```python
from build123d import *

# Parameters (mm, degrees)
SKETCH_5_W               = 17.572810229
SKETCH_5_H               = 5
EXTRUDE_1_DEPTH          = 6
CUT_EXTRUDE_1_DEPTH      = 50.115553238
CUT_EXTRUDE_1_DEPTH_BACK = 50.115553238
SKETCH_6_R               = 1.5
CUT_EXTRUDE_2_DEPTH      = 50.168435707
CUT_EXTRUDE_2_DEPTH_BACK = 50.168435707
SKETCH_7_R               = 1.5


with BuildPart() as part:
    # 草图5 → 凸台-拉伸1 (new body)
    with BuildSketch(Plane.XY):
        with Locations((-39.757750763, 1.95)):
            Rectangle(SKETCH_5_W, SKETCH_5_H)
    extrude(amount=EXTRUDE_1_DEPTH)

    # 草图6 → 切除-拉伸1 (cut, two sides: drawn at the far end of the back side and taken through both)
    with BuildSketch(Plane.XY.offset(6).offset(-CUT_EXTRUDE_1_DEPTH_BACK)):
        with Locations((-37.544155877, 1.95)):
            Circle(SKETCH_6_R)
        with Locations((-44.544155877, 1.95)):
            Circle(SKETCH_6_R)
    extrude(amount=CUT_EXTRUDE_1_DEPTH + CUT_EXTRUDE_1_DEPTH_BACK, mode=Mode.SUBTRACT)

    # 草图7 → 切除-拉伸2 (cut, two sides: drawn at the far end of the back side and taken through both)
    with BuildSketch(Plane.XZ.offset(0.55).offset(-CUT_EXTRUDE_2_DEPTH_BACK)):
        with Locations((-40.971345648, 3)):
            Circle(SKETCH_7_R)
        with Locations((-33.971345648, 3)):
            Circle(SKETCH_7_R)
    extrude(amount=CUT_EXTRUDE_2_DEPTH + CUT_EXTRUDE_2_DEPTH_BACK, mode=Mode.SUBTRACT)


solid = part.part
```
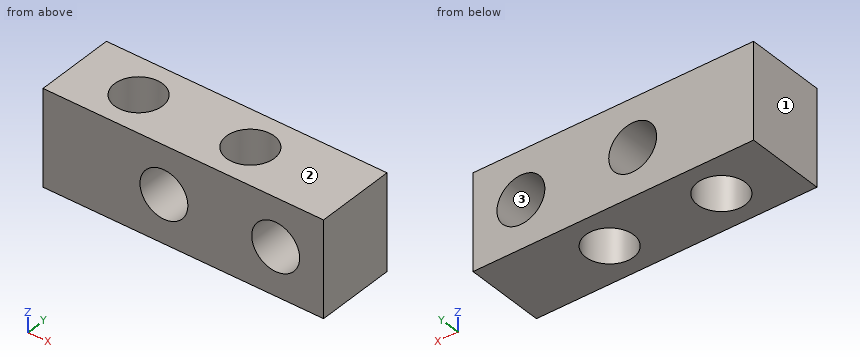
Can you work these out from the model? Positions are in its coordinate system, mm. Face numbers are marked on the shaded views. Round coordinates to 2 decimals unless told otherwise and drop trailing zeros. Loops run counter-clockwise (first coordinate to the right, second up) from the corner with the lowest first, then second, coordinate; pieces in that order, holes last.
Item 1: Will this pin go through, and if not, where does the flat tip stop? pin 1 Ø2.5 at (x, z) = (-33.97, 3) entering from +Y.
Item 2: Suppose I cut it at C-C, the plane x = -40. Write out the boundary of the cut face in (y, z), then the cut area to 3 significant figures.
Item 3: If we mould it in two halves opening along X, with no side actions, what happens to the marked faces 1, 2 and 3? For each: +X half, -X half, draft (parallel to the pull), parting line (faces both ways), or undercut.
Item 4: Suppose I cut it at A-A, the plane z = 3. Write out the boundary of the cut face in (x, y), then the cut area to 3 significant figures.
Item 5: Suppose I cut it at B-B, the plane y = 1.95. Write out the boundary of the cut face in (x, z).
Item 6: Suppose I cut it at D-D, the plane z = 4.75. Write out the boundary of the cut face in (x, y), then the cut area to 3 significant figures.
Item 7: Please list where these lines run through material, in increasing order: L1, parallel to X at y = 3.75, z = 3; L2, parallel to Y at x = -37.5, z = 3.85; L3, parallel to X at y = 3.55, z = 2.7.
Reported:
1. pin 1: passes through
2. outline: (-0.55, 0) - (4.45, 0) - (4.45, 1.86) - (-0.55, 1.86) - close; (-0.55, 4.14) - (4.45, 4.14) - (4.45, 6) - (-0.55, 6) - close
2. area: 18.6 mm2
3. face 1: -X half
3. face 2: draft
3. face 3: undercut
4. outline: (-48.54, -0.55) - (-42.47, -0.55) - (-42.47, 4.45) - (-48.54, 4.45) - close; (-39.47, -0.55) - (-35.47, -0.55) - (-35.47, 4.45) - (-39.47, 4.45) - close; (-32.47, -0.55) - (-30.97, -0.55) - (-30.97, 4.45) - (-32.47, 4.45) - close; hole circle Ø3 at (-44.54, 1.95); hole circle Ø3 at (-37.54, 1.95)
4. area: 43.7 mm2
5. outline: (-48.54, 0) - (-46.04, 0) - (-46.04, 6) - (-48.54, 6) - close; (-43.04, 0) - (-39.04, 0) - (-39.04, 6) - (-43.04, 6) - close; (-36.04, 0) - (-30.97, 0) - (-30.97, 6) - (-36.04, 6) - close; hole circle Ø3 at (-40.97, 3); hole circle Ø3 at (-33.97, 3)
6. outline: (-48.54, -0.55) - (-30.97, -0.55) - (-30.97, 4.45) - (-48.54, 4.45) - close; hole circle Ø3 at (-44.54, 1.95); hole circle Ø3 at (-37.54, 1.95)
6. area: 73.7 mm2
7. L1: x = -48.54 to -42.47, -39.47 to -35.47, -32.47 to -30.97
7. L2: y = -0.55 to 0.45, 3.45 to 4.45
7. L3: x = -48.54 to -42.44, -39.5 to -35.44, -32.5 to -30.97
